For this review, take the finished solid that the model builds, in its own axes (mm). Face numbers are marked on the shaded views. A direction names the side the tool comes from. Round coordinates to 2 decimals unless told otherwise and drop trailing zeros. Loops run counter-clockwise (first coordinate to the right, second up) from the corner with the lowest first, then second, coordinate; pieces in that order, holes last. Notation, with made-up numbers: (29, 72) -> (86, 72) arc R31 cw to (86, 109) -> close; hole circle Ø10 at (58, -26). An arc over 180 degrees is marked (long way). One line per question, with ' | ' between items. Start each with the question number.
1. Consider section C-C (y = -12). Write out the cut boundary in (x, z), and give its area (3 significant figures).
2. For the marked faces 1, 2, 3, 4 and 5, list the 3-axis set-ups (+Z, -Z, +X, -X, +Y, -Y) from which the entire face can be reached by the end or side of a thin tool; tool diameter is ignored.
3. Draft analysis for pull direction Y (two halves, no side actions). For the marked faces 6, 7 and 8, state which applies: pulls with the +Y half, pulls with the -Y half, needs draft (parallel to the pull), parting line crosses it, or undercut.
4. Consider section B-B (x = -31). Write out the cut boundary in (y, z).
5. Consider section A-A (z = 10). Count the separate pieces of the cut face and the enclosed holes in it, and give its area (3 significant figures).
6. For pin 1 Ø5 at (x, y) = (23, 12.5) entering from +Z; pin 2 Ø3 at (y, z) = (7, 3) entering from -X; pin 3 Ø6 at (y, z) = (-9, 10.5) entering from +X; pin 4 Ø3 at (x, z) = (39.4, 10) entering from +Y, all flat-tipped, find the tip position at first contact; note any pin that passes through.
7. Consider section D-D (z = 16). Write out the cut boundary in (x, y).
8. Wall thickness on line 1 along X through (y, z) = (-18.75, 10); line 2 along X through (y, z) = (-13.5, 11.25); line 3 along X through (y, z) = (18, 13): over which ranges is each line inside the solid? List them lowest first.
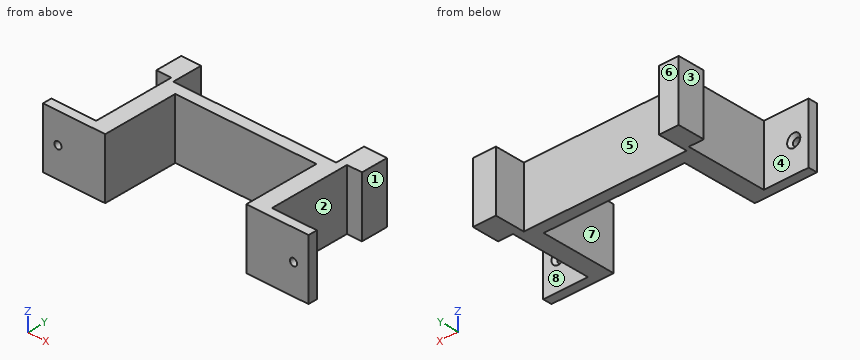
```python
from build123d import *

# Parameters (mm, degrees)
SKETCH1_W                                       = 68.8
SKETCH1_H                                       = 39
BOSS_EXTRUDE1_DEPTH                             = 20
SKETCH2_W                                       = 47.2
SKETCH2_H                                       = 25.2
SKETCH2_W_2                                     = 54.5
SKETCH2_H_2                                     = 10
CUT_EXTRUDE1_DEPTH                              = 50
SKETCH3_W                                       = 5
SKETCH3_H                                       = 30
CUT_EXTRUDE2_DEPTH                              = 50
SKETCH4_W                                       = 20
SKETCH4_H                                       = 3
BOSS_EXTRUDE2_DEPTH                             = 15
SKETCH5_W                                       = 20
SKETCH5_H                                       = 3
BOSS_EXTRUDE3_DEPTH                             = 15
CSK_FOR_M2_FLAT_HEAD_MACHINE_SCREW1_D           = 2.4
CSK_FOR_M2_FLAT_HEAD_MACHINE_SCREW1_CSINK_D     = 4.4
CSK_FOR_M2_FLAT_HEAD_MACHINE_SCREW1_CSINK_ANGLE = 90
CSK_FOR_M2_FLAT_HEAD_MACHINE_SCREW2_D           = 2.4
CSK_FOR_M2_FLAT_HEAD_MACHINE_SCREW2_CSINK_D     = 4.4
CSK_FOR_M2_FLAT_HEAD_MACHINE_SCREW2_CSINK_ANGLE = 90


with BuildPart() as part:
    # Sketch1 → Boss-Extrude1 (new body)
    with BuildSketch(Plane.XY):
        Rectangle(SKETCH1_W, SKETCH1_H)
    extrude(amount=BOSS_EXTRUDE1_DEPTH)

    # Sketch2 → Cut-Extrude1 (cut)
    with BuildSketch(Plane.XY.offset(20)):
        with Locations((0, -6.9)):
            Rectangle(SKETCH2_W, SKETCH2_H)
        with Locations((-0.54, 14.5)):
            Rectangle(SKETCH2_W_2, SKETCH2_H_2)
    extrude(amount=-CUT_EXTRUDE1_DEPTH, mode=Mode.SUBTRACT)

    # Sketch3 → Cut-Extrude2 (cut)
    with BuildSketch(Plane.XY.offset(20)):
        with Locations((-31.9, -4.5)):
            Rectangle(SKETCH3_W, SKETCH3_H)
        with Locations((31.9, -4.5)):
            Rectangle(SKETCH3_W, SKETCH3_H)
    extrude(amount=-CUT_EXTRUDE2_DEPTH, mode=Mode.SUBTRACT)

    # Sketch4 → Boss-Extrude2 (add)
    with BuildSketch(Plane.ZY.offset(29.4)):
        with Locations((10, -18)):
            Rectangle(SKETCH4_W, SKETCH4_H)
    extrude(amount=BOSS_EXTRUDE2_DEPTH)

    # Sketch5 → Boss-Extrude3 (add)
    with BuildSketch(Plane(origin=(29.4, 0, 0), x_dir=(0, 0, -1), z_dir=(1, 0, 0))):
        with Locations((-10, -18)):
            Rectangle(SKETCH5_W, SKETCH5_H)
    extrude(amount=BOSS_EXTRUDE3_DEPTH)

    # CSK for M2 Flat Head Machine Screw1 (through all)
    with Locations(Plane(origin=(0, -16.5, 0), x_dir=(1, 0, 0), z_dir=(0, 1, 0))):
        with Locations((-39.4, -10)):
            CounterSinkHole(CSK_FOR_M2_FLAT_HEAD_MACHINE_SCREW1_D / 2, CSK_FOR_M2_FLAT_HEAD_MACHINE_SCREW1_CSINK_D / 2, counter_sink_angle=CSK_FOR_M2_FLAT_HEAD_MACHINE_SCREW1_CSINK_ANGLE)

    # CSK for M2 Flat Head Machine Screw2 (through all)
    with Locations(Plane(origin=(0, -16.5, 0), x_dir=(1, 0, 0), z_dir=(0, 1, 0))):
        with Locations((39.4, -10)):
            CounterSinkHole(CSK_FOR_M2_FLAT_HEAD_MACHINE_SCREW2_D / 2, CSK_FOR_M2_FLAT_HEAD_MACHINE_SCREW2_CSINK_D / 2, counter_sink_angle=CSK_FOR_M2_FLAT_HEAD_MACHINE_SCREW2_CSINK_ANGLE)


solid = part.part
```
Answer block:
1) outline: (-29.4, 0) -> (-23.6, 0) -> (-23.6, 20) -> (-29.4, 20) -> close; (23.6, 0) -> (29.4, 0) -> (29.4, 20) -> (23.6, 20) -> close | area: 232 mm2
2) face 1: +Z, -Z, +X, +Y | face 2: +Z, -Z, +X | face 3: +Z, -Z, -X, +Y | face 4: +Z, -Z, -X | face 5: +Z, -Z, +Y
3) face 6: pulls with the +Y half | face 7: needs draft | face 8: undercut
4) outline: (-19.5, 0) -> (-16.5, 0) -> (-16.5, 20) -> (-19.5, 20) -> close; (10.5, 0) -> (19.5, 0) -> (19.5, 20) -> (10.5, 20) -> close
5) separate pieces: 3 | enclosed holes: 0 | area: 722 mm2
6) pin 1: passes through | pin 2: stops at x = -29.4 | pin 3: stops at x = 29.4 | pin 4: stops at y = -17.2
7) outline: (-44.4, -19.5) -> (-23.6, -19.5) -> (-23.6, 5.7) -> (23.6, 5.7) -> (23.6, -19.5) -> (44.4, -19.5) -> (44.4, -16.5) -> (29.4, -16.5) -> (29.4, 10.5) -> (34.4, 10.5) -> (34.4, 19.5) -> (26.71, 19.5) -> (26.71, 9.5) -> (-27.79, 9.5) -> (-27.79, 19.5) -> (-34.4, 19.5) -> (-34.4, 10.5) -> (-29.4, 10.5) -> (-29.4, -16.5) -> (-44.4, -16.5) -> close
8) line 1: x = -44.4 to -40.6, -38.2 to -23.6, 23.6 to 38.2, 40.6 to 44.4 | line 2: x = -29.4 to -23.6, 23.6 to 29.4 | line 3: x = -34.4 to -27.79, 26.71 to 34.4
